Geometry: final body of the model. Coordinates: model frame, mm. Face numbers are marked on the shaded views. A direction names the side the tool comes from. Coordinates: 2 decimals unless noted, no trailing zeros. Order: outer loops, then holes, each group sorted by start corner. A loop starts at its lowest first (then second) coordinate and runs counter-clockwise, first axis right, second up. Notation, with made-up numbers: M -33,-21.75 L 7,-21.75 A30 cw 7,7.25 Z; hole C 23,18.5 d7. An arc over 180 degrees is marked long. One line per question, with ' | ' between items.
from build123d import *

# Parameters (mm, degrees)
F0_W      = 133
F0_H      = 40
F1_DEPTH  = 17
F2_W      = 26
F2_H      = 5
F3_DEPTH  = 15
F4_R      = 1
F5_R      = 0.5
F6_R      = 5
F7_R      = 3
F10_DEPTH = 15


with BuildPart() as f1:
    # F0 (on Top) → F1 (new body)
    with BuildSketch(Plane.XY):
        Rectangle(F0_W, F0_H)
    extrude(amount=F1_DEPTH)

    # F2 (on face) → F3 (cut)
    with BuildSketch(Plane.XY.offset(17)):
        with Locations((-16.5, 14.5)):
            Rectangle(F2_W, F2_H)
        with Locations((16.5, 14.5)):
            Rectangle(F2_W, F2_H)
        with Locations((49.5, 14.5)):
            Rectangle(F2_W, F2_H)
        Polygon((-49.5, -15.5), (-42.5, -15.5), (-42.5, 5.5), (-63.5, 5.5), (-63.5, -15.5), (-56.5, -15.5), align=None)
        with BuildLine():
            ThreePointArc((-17.5, -5), (-33.2008771255, 3.2158383626), (-31, -14.3674969976))
            ThreePointArc((-31, -14.3674969976), (-27.5, -15), (-24, -14.3674969976))
            ThreePointArc((-24, -14.3674969976), (-19.2841616374, -10.7008771255), (-17.5, -5))
        make_face()
        with BuildLine():
            ThreePointArc((34.5, -5), (18.7991228745, 3.2158383626), (21, -14.3674969976))
            ThreePointArc((21, -14.3674969976), (24.5, -15), (28, -14.3674969976))
            ThreePointArc((28, -14.3674969976), (32.7158383626, -10.7008771255), (34.5, -5))
        make_face()
        with BuildLine():
            ThreePointArc((48, -16.4782402832), (51.5, -17), (55, -16.4782402832))
            ThreePointArc((55, -16.4782402832), (61.143650761, -12.1414284285), (63.5, -5))
            ThreePointArc((63.5, -5), (44.3585715715, 4.643650761), (48, -16.4782402832))
        make_face()
        Polygon((-13, -14.9595), (-5, -14.9595), (-1.5, -14.9595), (-1.5, 4.95908), align=None)
        Polygon((-1.5, 4.95908), (-1.5, -14.9595), (2, -14.9595), (10, -14.9595), align=None)
        with Locations((-49.5, 14.5)):
            Rectangle(F2_W, F2_H)
        Polygon((-45.7240516597, -20), (-49.5, -15.5), (-56.5, -15.5), (-60.2759483403, -20), align=None)
        with BuildLine():
            Line((-31, -14.3674969976), (-35.7262311919, -20))
            Line((-35.7262311919, -20), (-19.2737688081, -20))
            Line((-19.2737688081, -20), (-24, -14.3674969976))
            ThreePointArc((-24, -14.3674969976), (-27.5, -15), (-31, -14.3674969976))
        make_face()
        Polygon((-5, -14.9595), (-9.2294816909, -20), (6.2294816909, -20), (2, -14.9595), (-1.5, -14.9595), align=None)
        with BuildLine():
            Line((21, -14.3674969976), (16.2737688081, -20))
            Line((16.2737688081, -20), (32.7262311919, -20))
            Line((32.7262311919, -20), (28, -14.3674969976))
            ThreePointArc((28, -14.3674969976), (24.5, -15), (21, -14.3674969976))
        make_face()
        with BuildLine():
            Line((45.0448927206, -20), (57.9551072794, -20))
            Line((57.9551072794, -20), (55, -16.4782402832))
            ThreePointArc((55, -16.4782402832), (51.5, -17), (48, -16.4782402832))
            Line((48, -16.4782402832), (45.0448927206, -20))
        make_face()
    extrude(amount=-F3_DEPTH, mode=Mode.SUBTRACT)

    # F4
    f4_edges = [f1.edges().sort_by_distance(p)[0] for p in [
        (21, -14.367497, 9.5),
        (28, -14.367497, 9.5),
        (55, -16.47824, 9.5),
        (57.955107, -20, 9.5),
        (45.044893, -20, 9.5),
        (48, -16.47824, 9.5),
        (32.726231, -20, 9.5),
        (16.273769, -20, 9.5),
        (6.229482, -20, 9.5),
        (2, -14.9595, 9.5),
        (-5, -14.9595, 9.5),
        (-9.229482, -20, 9.5),
        (-24, -14.367497, 9.5),
        (-19.273769, -20, 9.5),
        (-31, -14.367497, 9.5),
        (-35.726231, -20, 9.5),
        (-56.5, -15.5, 9.5),
        (-60.275948, -20, 9.5),
        (-49.5, -15.5, 9.5),
        (-45.724052, -20, 9.5),
    ]]
    fillet(f4_edges, radius=F4_R)

    # F5
    f5_edges = [f1.edges().sort_by_distance(p)[0] for p in [
        (-1.5, 4.95908, 9.5),
        (-13, -14.9595, 9.5),
        (10, -14.9595, 9.5),
    ]]
    fillet(f5_edges, radius=F5_R)

    # F6
    f6_edges = [f1.edges().sort_by_distance(p)[0] for p in [
        (-66.5, -20, 8.5),
        (-66.5, 20, 8.5),
        (66.5, -20, 8.5),
        (66.5, 20, 8.5),
    ]]
    fillet(f6_edges, radius=F6_R)

    # F7
    f7_edges = [f1.edges().sort_by_distance(p)[0] for p in [
        (-42.5, 5.5, 9.5),
        (-63.5, 5.5, 9.5),
        (-63.5, -15.5, 9.5),
        (-42.5, -15.5, 9.5),
    ]]
    fillet(f7_edges, radius=F7_R)

    # F9 (on face) → F10 (cut)
    with BuildSketch(Plane(origin=(0, 0, 0), x_dir=(1, 0, 0), z_dir=(0, 0, -1))):
        with BuildLine():
            Line((-39.5, -9), (-2.6310750496, -9))
            Line((-2.6310750496, -9), (-16.2277130067, 14.5500626852))
            Line((-16.2277130067, 14.5500626852), (-14.6648491969, 17))
            Line((-14.6648491969, 17), (-17.8748458336, 17))
            Line((-17.8748458336, 17), (-19.4071963049, 15.1738158207))
            ThreePointArc((-19.4071963049, 15.1738158207), (-15.7908914081, 10.6477230794), (-14.5, 5))
            ThreePointArc((-14.5, 5), (-24.9504902432, -7.747548784), (-39.5, 0))
            Line((-39.5, 0), (-39.5, -9))
        make_face()
        with BuildLine():
            Line((13.1582028158, 14.4296675288), (-0.3689249504, -9))
            Line((-0.3689249504, -9), (46.1148351929, -9))
            ThreePointArc((46.1148351929, -9), (40.2858667229, -4.9620888795), (36.962962963, 1.3020878615))
            ThreePointArc((36.962962963, 1.3020878615), (17.2280826359, -5.7758627427), (16.4071963049, 15.1738158207))
            Line((16.4071963049, 15.1738158207), (14.8748458336, 17))
            Line((14.8748458336, 17), (11.7246036518, 17))
            Line((11.7246036518, 17), (13.1582028158, 14.4296675288))
        make_face()
        with BuildLine():
            ThreePointArc((66.5, 5), (63.8648184804, -3.4918351342), (56.8851648071, -9))
            Line((56.8851648071, -9), (66.5, -9))
            Line((66.5, -9), (66.5, 5))
        make_face()
    extrude(amount=-F10_DEPTH, mode=Mode.SUBTRACT)


solid = f1.part
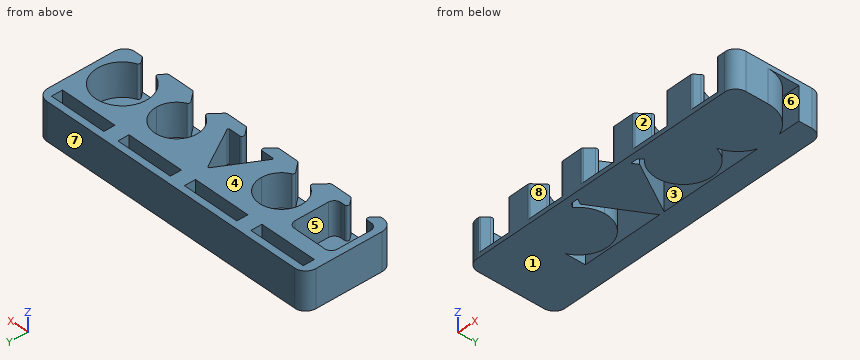
1. Section D-D, the plane x = 51.5. Output: boundary loops of the cut face in (y, z), and give its area (3 significant figures).
Response values:
outline: M -20,0 L 20,0 L 20,17 L 17,17 L 17,2 L 12,2 L 12,17 L 7,17 L 7,2 L -20,2 Z | area: 200 mm^2
2. Section B-B, the plane y = 13.5. Output: boundary loops of the cut face in (x, z).
Response values:
outline: M -66.5,0 L 66.5,0 L 66.5,17 L 62.5,17 L 62.5,2 L 36.5,2 L 36.5,17 L 29.5,17 L 29.5,2 L 3.5,2 L 3.5,17 L -3.5,17 L -3.5,2 L -29.5,2 L -29.5,17 L -36.5,17 L -36.5,2 L -62.5,2 L -62.5,17 L -66.5,17 Z
3. Section C-C, the plane z = 6.5. Give the number of separate pieces and of enclosed holes in the cut face, and give its area (3 significant figures).
Response values:
separate pieces: 1 | enclosed holes: 6 | area: 2,240 mm^2
4. Section A-A, the plane x = -27.5. Output: boundary loops of the cut face in (y, z).
Response values:
outline: M -20,0 L 8,0 L 8,15 L 9,15 L 9,0 L 20,0 L 20,17 L 17,17 L 17,2 L 12,2 L 12,17 L 5,17 L 5,2 L -20,2 Z
5. Pin query (flat end, axial travel): P1, Ø4.5, axis at x = -52, z = 10, coming from the -Y side; P2, Ø4.5, axis at x = -21.5, z = 10.5, coming from the -Y side. Return the tip coordinate at first contact, or that it passes through.
Response values:
P1: stops at y = 5.5 | P2: stops at y = -19.9
6. Draft query along Y for the marked faces 6, 7 and 8. Return one class per face: pulls with the +Y half, pulls with the -Y half, needs draft (parallel to the pull), parting line crosses it, or undercut.
Response values:
face 6: undercut | face 7: pulls with the +Y half | face 8: pulls with the -Y half
7. Access query for the marked faces 1, 2, 3, 4 and 5. Directions: +Z, -Z, +X, -X, +Y, -Y. A direction counts if a zero-diameter tool reaches every point of the face in a straight line with its end or side. Return the directions, or none.
Response values:
face 1: -Z, +X, -X, +Y, -Y | face 2: +Z, -Y | face 3: -Z | face 4: +Z, +X, -X, +Y, -Y | face 5: +Z
8. Material intervals for line 1 (Y direction, x = 25, z = 7.75); line 2 (Y direction, x = 8, z = 3); line 3 (Y direction, x = -49.5, z = 10), sorted ascending. Write a range as [from, to].
Response values:
line 1: y = [4.99, 7.99], [9, 12], [17, 20] | line 2: y = [-20, -14.96], [-11.5, -5.5], [9, 12], [17, 20] | line 3: y = [5.5, 12], [17, 20]
